CAD build for the part. Positions are in the model's coordinates, mm. A direction names the side the tool comes from. Give positions to 0.01 mm unless a question says otherwise; leave off trailing zeros. Order: outer loops, then holes, each group sorted by start corner. A loop starts at its lowest first (then second) coordinate and runs counter-clockwise, first axis right, second up.
Item 1: Band-saw the part on A-A on x = 0. Give the cut face in (y, z), plus the area to 3 significant figures.
Item 2: Band-saw the part on C-C on y = 4. Give the cut face in (x, z).
Item 3: Wall check: L1, parallel to Y at x = 0, z = 3.75; L2, parallel to X at y = 9, z = -1.5; L3, parallel to Y at x = -17, z = -4.25. Give the ranges that are in metal, low to high.
Item 4: Two-plate mould, pull along Y, no slides. Class faces 1 (the flat face through (-17, 0, 6.35)), 2 (the cylindrical face through (15.12, 11.59, 0.11)), 3 (the flat face through (-17, 6, 7.938)): released by +Y, released by -Y, zero draft, split by the parting line, or undercut.
Item 5: Which spindle directions (+Z, -Z, +X, -X, +Y, -Y) get a long thin tool onto all of the face, cutting with end or side? Do faces 4 (the flat face through (-5, -16, 6.35)), 5 (the flat face through (-9, 14, -6.35)). Say none if no direction does.
Item 6: Flat gauge pins, fed straight in: P1, Ø0.6, axis at x = -15.5, y = 6.5, coming from the -Z side; P2, Ø8, axis at y = -5.5, z = -3.5, coming from the +X side; P3, Ø3, axis at x = -4, z = -3, coming from the +Y side; P4, Ø8, axis at y = 3.5, z = -6.5, coming from the +X side. Where does each tip first touch, or does it go through?
```python
from build123d import *

# Parameters (mm, degrees)
F0_W     = 1.5875
F0_H     = 15.875
F2_R     = 1.13983
F3_DEPTH = 6.35


with BuildPart() as f1:
    # F0 (on Front) → F1 (revolve)
    with BuildSketch(Plane.XZ):
        with Locations((-18.25625, 0)):
            Rectangle(F0_W, F0_H)
    revolve(axis=Axis((0, 0, 36.088426), (0, 0, 1)))

    # F2 (on Top) → F3 (join, symmetric)
    with BuildSketch(Plane.XY):
        with Locations((17.01483, 0)):
            Circle(F2_R)
        with Locations((16.643015, 3.537582)):
            Circle(F2_R)
        with Locations((15.543821, 6.920555)):
            Circle(F2_R)
        with Locations((13.765287, 10.001066)):
            Circle(F2_R)
        with Locations((11.385144, 12.644483)):
            Circle(F2_R)
        with Locations((8.507415, 14.735275)):
            Circle(F2_R)
        with Locations((5.257872, 16.182065)):
            Circle(F2_R)
        with Locations((1.778534, 16.921621)):
            Circle(F2_R)
        with Locations((-1.778534, 16.921621)):
            Circle(F2_R)
        with Locations((-5.257872, 16.182065)):
            Circle(F2_R)
        with Locations((-8.507415, 14.735275)):
            Circle(F2_R)
        with Locations((-11.385144, 12.644483)):
            Circle(F2_R)
        with Locations((-13.765287, 10.001066)):
            Circle(F2_R)
        with Locations((-15.543821, 6.920555)):
            Circle(F2_R)
        with Locations((-16.643015, 3.537582)):
            Circle(F2_R)
        with Locations((-17.01483, 0)):
            Circle(F2_R)
        with Locations((-16.643015, -3.537582)):
            Circle(F2_R)
        with Locations((-15.543821, -6.920555)):
            Circle(F2_R)
        with Locations((-13.765287, -10.001066)):
            Circle(F2_R)
        with Locations((-11.385144, -12.644483)):
            Circle(F2_R)
        with Locations((-8.507415, -14.735275)):
            Circle(F2_R)
        with Locations((-5.257872, -16.182065)):
            Circle(F2_R)
        with Locations((-1.778534, -16.921621)):
            Circle(F2_R)
        with Locations((1.778534, -16.921621)):
            Circle(F2_R)
        with Locations((5.257872, -16.182065)):
            Circle(F2_R)
        with Locations((8.507415, -14.735275)):
            Circle(F2_R)
        with Locations((11.385144, -12.644483)):
            Circle(F2_R)
        with Locations((13.765287, -10.001066)):
            Circle(F2_R)
        with Locations((15.543821, -6.920555)):
            Circle(F2_R)
        with Locations((16.643015, -3.537582)):
            Circle(F2_R)
    extrude(amount=F3_DEPTH, both=True)


solid = f1.part
```
The answers:
1. outline: (-19.05, -7.94) - (-17.46, -7.94) - (-17.46, 7.94) - (-19.05, 7.94) - close; (17.46, -7.94) - (19.05, -7.94) - (19.05, 7.94) - (17.46, 7.94) - close
1. area: 50.4 mm2
2. outline: (-18.63, -7.94) - (-17, -7.94) - (-17, -6.35) - (-15.6, -6.35) - (-15.6, 6.35) - (-17, 6.35) - (-17, 7.94) - (-18.63, 7.94) - close; (15.6, -6.35) - (17, -6.35) - (17, -7.94) - (18.63, -7.94) - (18.63, 7.94) - (17, 7.94) - (17, 6.35) - (15.6, 6.35) - close
3. L1: y = -19.05 to -17.46, 17.46 to 19.05
3. L2: x = -16.79 to -14.96, -14.31 to -13.22, 13.22 to 14.31, 14.96 to 16.79
3. L3: y = -8.6 to -2.46, -1.14 to 1.14, 2.46 to 8.6
4. face 1: undercut
4. face 2: split by the parting line
4. face 3: zero draft
5. face 4: +Z
5. face 5: -Z
6. P1: stops at z = -6.35
6. P2: stops at x = 18.99
6. P3: stops at y = 18.89
6. P4: stops at x = 19.05
